Can you work these out from the model? Positions are in its coordinate system, mm. A direction names the side the tool comes from. Give positions to 0.01 mm unless a question says otherwise; leave off trailing zeros. Loops run counter-clockwise (first coordinate to the right, second up) from the corner with the lowest first, then second, coordinate; pieces in that order, holes last. Notation, with made-up numbers: (9.25, 71) -> (50.25, 71) arc R9 cw to (50.25, 88) -> close; hole circle Ø10 at (22.25, -38.75). An arc over 180 degrees is marked (long way). Use CSV: the item, a comma, the result in double quotes.
from build123d import *

# Parameters (mm, degrees)
SALIENTE_EXTRUIR1_DEPTH = 5
CROQUIS2_R              = 2
CROQUIS2_R_2            = 4.05
CROQUIS2_R_3            = 1.5
CROQUIS2_R_4            = 5.5
CORTAR_EXTRUIR1_DEPTH   = 10


with BuildPart() as part:
    # Croquis1 → Saliente-Extruir1 (new body)
    with BuildSketch(Plane.XY):
        with BuildLine():
            Line((110, 30), (80, 30))
            ThreePointArc((80, 30), (72.928932188, 27.071067812), (70, 20))
            Line((70, 20), (70, 10))
            ThreePointArc((70, 10), (67.071067812, 2.928932188), (60, 0))
            Line((60, 0), (10, 0))
            ThreePointArc((10, 0), (2.928932188, 2.928932188), (0, 10))
            Line((0, 10), (0, 110))
            ThreePointArc((0, 110), (2.928932188, 117.071067812), (10, 120))
            Line((10, 120), (110, 120))
            ThreePointArc((110, 120), (117.071067812, 117.071067812), (120, 110))
            Line((120, 110), (120, 40))
            ThreePointArc((120, 40), (117.071067812, 32.928932188), (110, 30))
        make_face()
    extrude(amount=SALIENTE_EXTRUIR1_DEPTH)

    # Croquis2 → Cortar-Extruir1 (cut)
    with BuildSketch(Plane.XY.offset(5)):
        with Locations((8, 112)):
            Circle(CROQUIS2_R)
        with Locations((8, 8)):
            Circle(CROQUIS2_R)
        with Locations((112, 8)):
            Circle(CROQUIS2_R)
        with Locations((112, 112)):
            Circle(CROQUIS2_R)
        with Locations((62, 8)):
            Circle(CROQUIS2_R)
        with Locations((24.9, 60)):
            Circle(CROQUIS2_R_2)
        with Locations((82.25, 80.423393759)):
            Circle(CROQUIS2_R_3)
        with Locations((97.75, 80.423393759)):
            Circle(CROQUIS2_R_3)
        with Locations((105.5, 67)):
            Circle(CROQUIS2_R_3)
        with Locations((97.75, 53.576606241)):
            Circle(CROQUIS2_R_3)
        with Locations((82.25, 53.576606241)):
            Circle(CROQUIS2_R_3)
        with Locations((74.5, 67)):
            Circle(CROQUIS2_R_3)
        with Locations((90, 60)):
            Circle(CROQUIS2_R_4)
    extrude(amount=-CORTAR_EXTRUIR1_DEPTH, mode=Mode.SUBTRACT)


solid = part.part
(1) If I drill on L1, parallel to X at y = 67, z = 2.2; L2, parallel to Y at x = 97.75, z = 2; L3, parallel to Y at x = 105.5, z = 3.5, over which ranges is the centre line in solid material (lowest first)? Write a range as from..to.
Answer sheet:
L1,"x = 0..73, 76..104, 107..120"
L2,"y = 30..52.08, 55.08..78.92, 81.92..120"
L3,"y = 30..65.5, 68.5..120"
(2) If we section it at D-D, the plane x = 112: Write out the boundary of the cut face in (y, z).
Answer sheet:
outline,"(30.2, 0) -> (110, 0) -> (110, 5) -> (30.2, 5) -> close; (114, 0) -> (119.8, 0) -> (119.8, 5) -> (114, 5) -> close"
(3) If we section it at C-C, the plane z = 1.1: Give the number of separate pieces and of enclosed holes in the cut face, then the cut area to 3 significant figures.
Answer sheet:
separate pieces,"1"
enclosed holes,"12"
area,"12,600 mm2"
(4) We'd pull the mould along X, two halves only. Please class faces 3 (the face through (35, 0, 2)), 4 (the face through (60.526, 9.352, 2.535)), 5 (the face through (67.15, 3.01, 2.46)): released by +X, released by -X, zero draft, split by the parting line, or undercut.
Answer sheet:
face 3,"zero draft"
face 4,"undercut"
face 5,"released by +X"
(5) If we section it at B-B, the plane y = 67: Write out the boundary of the cut face in (x, z).
Answer sheet:
outline,"(0, 0) -> (73, 0) -> (73, 5) -> (0, 5) -> close; (76, 0) -> (104, 0) -> (104, 5) -> (76, 5) -> close; (107, 0) -> (120, 0) -> (120, 5) -> (107, 5) -> close"
(6) If we section it at A-A, the plane x = 97.75: Write out the boundary of the cut face in (y, z).
Answer sheet:
outline,"(30, 0) -> (52.08, 0) -> (52.08, 5) -> (30, 5) -> close; (55.08, 0) -> (78.92, 0) -> (78.92, 5) -> (55.08, 5) -> close; (81.92, 0) -> (120, 0) -> (120, 5) -> (81.92, 5) -> close"
(7) Will these pins go through, and if not, where does the flat tip stop? pin 1 Ø3 at (x, y) = (112, 112) entering from +Z (1 decimal); pin 2 Ø1.5 at (y, z) = (16.5, 1.5) entering from +X.
Answer sheet:
pin 1,"passes through"
pin 2,"stops at x = 70"
(8) Which directions (+Z, -Z, +X, -X, +Y, -Y) give clear straight access to the entire face, cutting with the end or side of a thin tool? Please do faces 1 (the face through (70, 15, 2)), 2 (the face through (61, 74, 0)).
Answer sheet:
face 1,"+Z, -Z, +X, -Y"
face 2,"-Z, +X, -X, +Y, -Y"
